```python
from build123d import *

# Parameters (mm, degrees)
F1_DEPTH = 6.985
F2_R     = 50.8
F3_SIZE  = 2.54


with BuildPart() as f1:
    # F0 (on Top) → F1 (new body)
    with BuildSketch(Plane.XY):
        with BuildLine():
            Line((-22.4686733496, -0.2763976852), (-11.3768203047, 20.0517258855))
            ThreePointArc((-11.3768203047, 20.0517258855), (-13.5749073132, 23.8222438401), (-14.5607446546, 28.0738925649))
            Line((-14.5607446546, 28.0738925649), (-30.3766020445, -0.9119497554))
            ThreePointArc((-30.3766020445, -0.9119497554), (-26.4666182407, -0.0469408196), (-22.4686733496, -0.2763976852))
        make_face()
        with BuildLine():
            ThreePointArc((14.5607446546, 28.0738925649), (13.5749073132, 23.8222438401), (11.3768203047, 20.0517258855))
            Line((11.3768203047, 20.0517258855), (22.4686733496, -0.2763976852))
            ThreePointArc((22.4686733496, -0.2763976852), (26.4666182407, -0.0469408196), (30.3766020445, -0.9119497554))
            Line((30.3766020445, -0.9119497554), (14.5607446546, 28.0738925649))
        make_face()
        with BuildLine():
            ThreePointArc((-4.8932738406, 15.4491171751), (-2.4756966767, 16.0153138069), (0, 16.2055345598))
            ThreePointArc((0, 16.2055345598), (2.4756966767, 16.0153138069), (4.8932738406, 15.4491171751))
            ThreePointArc((4.8932738406, 15.4491171751), (8.4542884153, 17.3007165459), (11.3768203047, 20.0517258855))
            ThreePointArc((11.3768203047, 20.0517258855), (13.5749073132, 23.8222438401), (14.5607446546, 28.0738925649))
            ThreePointArc((14.5607446546, 28.0738925649), (14.5939319698, 28.6415154708), (14.605, 29.21))
            ThreePointArc((14.605, 29.21), (-0.5684845292, 43.8039319698), (-14.5607446546, 28.0738925649))
            ThreePointArc((-14.5607446546, 28.0738925649), (-13.5749073132, 23.8222438401), (-11.3768203047, 20.0517258855))
            ThreePointArc((-11.3768203047, 20.0517258855), (-8.4542884153, 17.3007165459), (-4.8932738406, 15.4491171751))
        make_face()
        with BuildLine():
            ThreePointArc((10.9855, 29.21), (7.7679215447, 21.4420784553), (0, 18.2245))
            ThreePointArc((0, 18.2245), (-7.7679215447, 36.9779215447), (10.9855, 29.21))
        make_face(mode=Mode.SUBTRACT)
        with BuildLine():
            Line((0, 16.2055345598), (0, 14.605))
            ThreePointArc((0, 14.605), (2.4827737857, 14.8175763219), (4.8932738406, 15.4491171751))
            ThreePointArc((4.8932738406, 15.4491171751), (2.4756966767, 16.0153138069), (0, 16.2055345598))
        make_face()
        with BuildLine():
            ThreePointArc((-4.8932738406, 15.4491171751), (-2.4827737857, 14.8175763219), (0, 14.605))
            Line((0, 14.605), (0, 16.2055345598))
            ThreePointArc((0, 16.2055345598), (-2.4756966767, 16.0153138069), (-4.8932738406, 15.4491171751))
        make_face()
        with BuildLine():
            ThreePointArc((0, 10.9855), (7.7679215447, 7.7679215447), (10.9855, 0))
            ThreePointArc((10.9855, 0), (10.6111781647, -2.84325662), (9.5137220733, -5.49275))
            Line((9.5137220733, -5.49275), (12.6483010223, -7.3025))
            ThreePointArc((12.6483010223, -7.3025), (14.0737844102, -5.2586429907), (15.82596486, -3.4868591339))
            ThreePointArc((15.82596486, -3.4868591339), (16.1103626721, -1.7537288685), (16.2055345598, 0))
            ThreePointArc((16.2055345598, 0), (13.0751189039, 9.5739550875), (4.8932738406, 15.4491171751))
            ThreePointArc((4.8932738406, 15.4491171751), (2.4827737857, 14.8175763219), (0, 14.605))
            Line((0, 14.605), (0, 10.9855))
        make_face()
        with BuildLine():
            ThreePointArc((-9.5137220733, -5.49275), (-9.5137220733, 5.49275), (0, 10.9855))
            Line((0, 10.9855), (0, 14.605))
            ThreePointArc((0, 14.605), (-2.4827737857, 14.8175763219), (-4.8932738406, 15.4491171751))
            ThreePointArc((-4.8932738406, 15.4491171751), (-14.0344046107, 8.1027672799), (-15.82596486, -3.4868591339))
            ThreePointArc((-15.82596486, -3.4868591339), (-14.0737844102, -5.2586429907), (-12.6483010223, -7.3025))
            Line((-12.6483010223, -7.3025), (-9.5137220733, -5.49275))
        make_face()
        with BuildLine():
            Line((12.6483010223, -7.3025), (9.5137220733, -5.49275))
            ThreePointArc((9.5137220733, -5.49275), (0, -10.9855), (-9.5137220733, -5.49275))
            Line((-9.5137220733, -5.49275), (-12.6483010223, -7.3025))
            ThreePointArc((-12.6483010223, -7.3025), (-11.5910106244, -9.5589333313), (-10.9326910194, -11.9622580412))
            ThreePointArc((-10.9326910194, -11.9622580412), (0, -16.2055345598), (10.9326910194, -11.9622580412))
            ThreePointArc((10.9326910194, -11.9622580412), (11.5910106244, -9.5589333313), (12.6483010223, -7.3025))
        make_face()
        with BuildLine():
            ThreePointArc((16.51, -26.2712611625), (13.5628030503, -23.3012052737), (11.5786636953, -19.6174038591))
            Line((11.5786636953, -19.6174038591), (-11.5786636953, -19.6174038591))
            ThreePointArc((-11.5786636953, -19.6174038591), (-13.5628030503, -23.3012052737), (-16.51, -26.2712611625))
            Line((-16.51, -26.2712611625), (16.51, -26.2712611625))
        make_face()
        with BuildLine():
            ThreePointArc((-10.9326910194, -11.9622580412), (-12.6318202681, -10.1516731175), (-14.0344046107, -8.1027672799))
            ThreePointArc((-14.0344046107, -8.1027672799), (-15.1075169447, -5.8636406894), (-15.82596486, -3.4868591339))
            ThreePointArc((-15.82596486, -3.4868591339), (-18.94125419, -1.4552631719), (-22.4686733496, -0.2763976852))
            ThreePointArc((-22.4686733496, -0.2763976852), (-26.4666182407, -0.0469408196), (-30.3766020445, -0.9119497554))
            ThreePointArc((-30.3766020445, -0.9119497554), (-38.1109843332, -21.6119702127), (-16.51, -26.2712611625))
            ThreePointArc((-16.51, -26.2712611625), (-13.5628030503, -23.3012052737), (-11.5786636953, -19.6174038591))
            ThreePointArc((-11.5786636953, -19.6174038591), (-10.9150771847, -17.1501459103), (-10.6916020445, -14.605))
            ThreePointArc((-10.6916020445, -14.605), (-10.7519991706, -13.2781419674), (-10.9326910194, -11.9622580412))
        make_face()
        with BuildLine():
            ThreePointArc((-14.3111020445, -14.605), (-35.9077802092, -17.44825662), (-15.7828799713, -9.11225))
            ThreePointArc((-15.7828799713, -9.11225), (-14.6854238798, -11.76174338), (-14.3111020445, -14.605))
        make_face(mode=Mode.SUBTRACT)
        with BuildLine():
            ThreePointArc((-10.9326910194, -11.9622580412), (-11.5910106244, -9.5589333313), (-12.6483010223, -7.3025))
            Line((-12.6483010223, -7.3025), (-14.0344046107, -8.1027672799))
            ThreePointArc((-14.0344046107, -8.1027672799), (-12.6318202681, -10.1516731175), (-10.9326910194, -11.9622580412))
        make_face()
        with BuildLine():
            Line((-14.0344046107, -8.1027672799), (-12.6483010223, -7.3025))
            ThreePointArc((-12.6483010223, -7.3025), (-14.0737844102, -5.2586429907), (-15.82596486, -3.4868591339))
            ThreePointArc((-15.82596486, -3.4868591339), (-15.1075169447, -5.8636406894), (-14.0344046107, -8.1027672799))
        make_face()
        with BuildLine():
            Line((14.0344046107, -8.1027672799), (12.6483010223, -7.3025))
            ThreePointArc((12.6483010223, -7.3025), (11.5910106244, -9.5589333313), (10.9326910194, -11.9622580412))
            ThreePointArc((10.9326910194, -11.9622580412), (12.6318202681, -10.1516731175), (14.0344046107, -8.1027672799))
        make_face()
        with BuildLine():
            ThreePointArc((15.82596486, -3.4868591339), (15.1075169447, -5.8636406894), (14.0344046107, -8.1027672799))
            ThreePointArc((14.0344046107, -8.1027672799), (12.6318202681, -10.1516731175), (10.9326910194, -11.9622580412))
            ThreePointArc((10.9326910194, -11.9622580412), (10.7433247351, -15.8330653708), (11.5786636953, -19.6174038591))
            ThreePointArc((11.5786636953, -19.6174038591), (13.5628030503, -23.3012052737), (16.51, -26.2712611625))
            ThreePointArc((16.51, -26.2712611625), (31.8149493097, -27.6747044316), (39.9016020445, -14.605))
            ThreePointArc((39.9016020445, -14.605), (37.2861688632, -6.2649572843), (30.3766020445, -0.9119497554))
            ThreePointArc((30.3766020445, -0.9119497554), (26.4666182407, -0.0469408196), (22.4686733496, -0.2763976852))
            ThreePointArc((22.4686733496, -0.2763976852), (18.94125419, -1.4552631719), (15.82596486, -3.4868591339))
        make_face()
        with BuildLine():
            ThreePointArc((36.2821020445, -14.605), (22.4533454246, -25.2161781647), (15.7828799713, -9.11225))
            ThreePointArc((15.7828799713, -9.11225), (28.1398586645, -3.9938218353), (36.2821020445, -14.605))
        make_face(mode=Mode.SUBTRACT)
        with BuildLine():
            ThreePointArc((15.82596486, -3.4868591339), (14.0737844102, -5.2586429907), (12.6483010223, -7.3025))
            Line((12.6483010223, -7.3025), (14.0344046107, -8.1027672799))
            ThreePointArc((14.0344046107, -8.1027672799), (15.1075169447, -5.8636406894), (15.82596486, -3.4868591339))
        make_face()
    extrude(amount=F1_DEPTH)

    # F2
    f2_edges = [f1.edges().sort_by_distance(p)[0] for p in [
        (-14.560745, 28.073893, 3.4925),
        (-30.376602, -0.91195, 3.4925),
        (16.51, -26.271261, 3.4925),
        (-16.51, -26.271261, 3.4925),
        (14.560745, 28.073893, 3.4925),
        (30.376602, -0.91195, 3.4925),
    ]]
    fillet(f2_edges, radius=F2_R)

    # F3
    f3_edges = [f1.edges().sort_by_distance(p)[0] for p in [
        (-37.972945, -21.858713, 0),
        (-37.972945, -21.858713, 6.985),
    ]]
    chamfer(f3_edges, length=F3_SIZE)


solid = f1.part
```
For this review, take the finished solid that the model builds, in its own axes (mm). A direction names the side the tool comes from. Coordinates: 2 decimals unless noted, no trailing zeros. Use one line per item in the form item = value. Start each with the question number.
1) Draft analysis for pull direction Y (two halves, no side actions). For faces 4 (the face through (-0.083, -25.019, 5.697)), 5 (the face through (-18.89, -1.48, 3.44)), 6 (the face through (-29.31, 2.47, 3.51)), state which applies: released by +Y, released by -Y, zero draft, split by the parting line, or undercut.
2) Take a section at A-A (y = 7). State how many separate pieces and enclosed holes the cut face has, plus the area to 3 significant figures.
3) For faces 1 (the face through (-20.78, 14.07, 1.29)), 2 (the face through (16.845, 10.03, 3.444)), 3 (the face through (13.42, -26.83, 3.51)), list the 3-axis set-ups (+Z, -Z, +X, -X, +Y, -Y) from which the entire face can be reached by the end or side of a thin tool; tool diameter is ignored.
4) For pin 1 (1 mm diameter, centred on x = 24.5, z = 3.5, fed in from -Y); pin 2 (4 mm diameter, centred on x = 24.5, y = 13.5, fed in from -Z); pin 3 (1 mm diameter, centred on x = -1.5, z = 4, fed in from -Y), all flat-tipped, find the tip position at first contact; note any pin that passes through.
5) To check wall thickness, follow probe 1 along Y at (x, z) = (19, 5.5); probe 2 along X at (y, z) = (-15, 0.5) (3 decimals); probe 3 along Y at (x, z) = (4, 2.25). State the ranges of each line that lie inside material, in increasing order. Write a range as from..to.
From the geometry:
q1.face_4 = released by -Y
q1.face_5 = undercut
q1.face_6 = released by +Y
q2.separate_pieces = 4
q2.enclosed_holes = 0
q2.area = 178 mm2
q3.face_1 = -Z, -X, +Y
q3.face_2 = +Z, -Z
q3.face_3 = +Z, -Z, -Y
q4.pin_1 = -29.21
q4.pin_2 = 2.28
q4.pin_3 = -26.27
q5.probe_1 = -26.9..-23.61, -5.6..-1.43, 6.08..17.74
q5.probe_2 = -37.855..-36.275, -14.318..-10.697, -6.133..6.133, 10.697..14.318, 36.275..37.855
q5.probe_3 = -25.98..-19.62, -15.7..-10.23, 10.23..18.98, 39.44..42.95
